Source: CAD feature listing. Evaluate the final solid. Frame: model axes, mm. A direction names the side the tool comes from. Give positions to 0.01 mm unless a question says otherwise; leave off trailing zeros. Order: outer loops, then holes, each group sorted by start corner. A loop starts at its lowest first (then second) coordinate and runs counter-clockwise, first axis right, second up. Notation, with made-up numbers: M -16.75,87 L 16.25,87 A28 ccw 16.25,117 Z; hole C -25.5,39.5 d1. An arc over 180 degrees is marked long. Answer in a Markdown table with one row per item. Add a question column.
(1) Material intervals for line 1 along Z through (x, y) = (5.4, 10); line 2 along Z through (x, y) = (10, 2); line 3 along Z through (x, y) = (12.5, -8), sorted ascending.
(2) Section query C-C, the plane x = 17.25. Return loops of the section in (y, z), plus the area to 3 significant figures.
(3) Mould query, pull axis Y, two halves, no side actions, for faces 3 (the face through (9.909, -3.715, -28.293)), 4 (the face through (10.48, 10.26, 0.83)), 5 (the face through (0, 0, 0)). Classes: pulls with the +Y half, pulls with the -Y half, needs draft (parallel to the pull), parting line crosses it, or undercut.
(4) Pin query (flat end, axial travel): P1, Ø8, axis at y = 8.5, z = -2.5, coming from the -X side; P2, Ø5, axis at x = 9, z = -20, coming from the -Y side; P3, Ø5, axis at x = 10, y = 21, coming from the -Z side. Return the tip coordinate at first contact, or that it passes through.
(5) Section query A-A, the plane y = 0. Return loops of the section in (x, z), plus the area to 3 significant figures.
(6) Section query B-B, the plane x = 11.75. Return loops of the section in (y, z), plus the area to 3 significant figures.
(7) Set-up query: faces 1 (the face through (19.779, 24.056, -7.576)), 2 (the face through (5.288, 5.043, -0.651)). Return all of +Z, -Z, +X, -X, +Y, -Y with unobstructed straight access to the full face (end or side cutting, diameter ignored); none if empty.
Autodesk Inventor part; units mm, degrees
ref_plane "YZ Plane" through (0, 0, 0) normal (1, 0, 0) x (0, 1, 0)
ref_plane "XZ Plane" through (0, 0, 0) normal (0, 1, 0) x (-1, 0, 0)
ref_plane "XY Plane" through (0, 0, 0) normal (0, 0, 1) x (1, 0, 0)
sketch "Эскиз1" plane through (0, 0, 0) normal (0, 0, 1) x (1, 0, 0)
  line L0 (0, 0) -> (20, 0)
  line L1 (0, 0) -> (0, 25)
  line L2 (0, 25) -> (3.5355, 28.5355)
  line L3 (20, 0) -> (20, 25)
  line L4 (20, 25) -> (16.4645, 28.5355)
  line L5 (16.4645, 28.5355) -> (3.5355, 28.5355)
  dimension "d0" = 20
  dimension "d1" = 25
  dimension "d2" = 5
  dimension "d3" = 135
  dimension "d4" = 5
  dimension "d5" = 135
revolve "Вращение1" add sketch "Эскиз1" angle 360 about axis through (0, 0, 0) along (1, 0, 0)
sketch "Эскиз2" plane through (0, 0, 0) normal (-1, 0, 0) x (0, 0, 1)
  line L0 (0, 0) -> (0, 10) construction
  dimension "d7" = 10
hole "Отверстие1" at (0, 10, 0) direction (1, 0, 0) diameter 10 depth 8 tip angle 118 countersink diameter 15 countersink angle 90
properties part number "711112"
Values follow:
| question | item | result |
|---|---|---|
| 1 | line 1 | z = -26.73 to -5, 5 to 26.73 |
| 1 | line 2 | z = -28.47 to 28.47 |
| 1 | line 3 | z = -27.39 to 27.39 |
| 2 | outline | C 0,0 d55.5 |
| 2 | area | 2,420 mm² |
| 3 | face 3 | parting line crosses it |
| 3 | face 4 | undercut |
| 3 | face 5 | needs draft |
| 4 | P1 | stops at x = 0.58 |
| 4 | P2 | stops at y = -22.54 |
| 4 | P3 | stops at z = -21.73 |
| 5 | outline | M 0,-25 L 3.54,-28.54 L 16.46,-28.54 L 20,-25 L 20,25 L 16.46,28.54 L 3.54,28.54 L 0,25 Z |
| 5 | area | 1,120 mm² |
| 6 | outline | C 0,0 d57.07 |
| 6 | area | 2,560 mm² |
| 7 | face 1 | +X |
| 7 | face 2 | -X |
